Can you work these out from the model? Positions are in its coordinate system, mm. A direction names the side the tool comes from. Give positions to 0.01 mm unless a question says otherwise; leave off trailing zeros. Loops run counter-clockwise (first coordinate to the right, second up) from the corner with the lowest first, then second, coordinate; pieces in that order, holes last.
from build123d import *

# Parameters (mm, degrees)
SKETCH_1_R          = 30
SKETCH_1_R_2        = 15.5
EXTRUDE_1_DEPTH     = 8
SKETCH_2_R          = 21
CUT_EXTRUDE_1_DEPTH = 4
SKETCH_3_R          = 19
CUT_EXTRUDE_2_DEPTH = 1
SKETCH_4_R          = 2.25
CUT_EXTRUDE_3_DEPTH = 44.17406629
SKETCH_5_R          = 3.5
CUT_EXTRUDE_4_DEPTH = 4
CHAMFER_1_SIZE      = 1.414


with BuildPart() as part:
    # 草图1 → 拉伸1 (new body)
    with BuildSketch(Plane.XY):
        Circle(SKETCH_1_R)
        Circle(SKETCH_1_R_2, mode=Mode.SUBTRACT)
    extrude(amount=EXTRUDE_1_DEPTH)

    # 草图2 → 切除-拉伸1 (cut)
    with BuildSketch(Plane.XY.offset(8)):
        Circle(SKETCH_2_R)
    extrude(amount=-CUT_EXTRUDE_1_DEPTH, mode=Mode.SUBTRACT)

    # 草图3 → 切除-拉伸2 (cut)
    with BuildSketch(Plane.XY.offset(4)):
        Circle(SKETCH_3_R)
    extrude(amount=-CUT_EXTRUDE_2_DEPTH, mode=Mode.SUBTRACT)

    # 草图4 → 切除-拉伸3 (cut, through all)
    with BuildSketch(Plane(origin=(0, 0, 0), x_dir=(-1, 0, 0), z_dir=(0, 0, -1))):
        with Locations((12.5, 21.650635095)):
            Circle(SKETCH_4_R)
        with Locations((-12.5, 21.650635095)):
            Circle(SKETCH_4_R)
        with Locations((-25, 0)):
            Circle(SKETCH_4_R)
        with Locations((-12.5, -21.650635095)):
            Circle(SKETCH_4_R)
        with Locations((12.5, -21.650635095)):
            Circle(SKETCH_4_R)
        with Locations((25, 0)):
            Circle(SKETCH_4_R)
    extrude(amount=-CUT_EXTRUDE_3_DEPTH, mode=Mode.SUBTRACT)

    # 草图5 → 切除-拉伸4 (cut)
    with BuildSketch(Plane(origin=(0, 0, 0), x_dir=(-1, 0, 0), z_dir=(0, 0, -1))):
        with Locations((-12.5, 21.650635095)):
            Circle(SKETCH_5_R)
        with Locations((-25, 0)):
            Circle(SKETCH_5_R)
        with Locations((-12.5, -21.650635095)):
            Circle(SKETCH_5_R)
        with Locations((12.5, -21.650635095)):
            Circle(SKETCH_5_R)
        with Locations((25, 0)):
            Circle(SKETCH_5_R)
        with Locations((12.5, 21.650635095)):
            Circle(SKETCH_5_R)
    extrude(amount=-CUT_EXTRUDE_4_DEPTH, mode=Mode.SUBTRACT)

    # 倒角1
    chamfer_1_edges = [part.edges().sort_by_distance(p)[0] for p in [
        (-30, 0, 0),
    ]]
    chamfer(chamfer_1_edges, length=CHAMFER_1_SIZE)


solid = part.part
(1) Will these pins go through, and if not, where does the flat tip stop? P1, Ø3.5, axis at x = 11.5, y = 22.5, coming from the -Z side; P2, Ø2, axis at x = -14.5, z = 2, coming from the -Y side; P3, Ø4, axis at x = 12, z = 4.5, coming from the +Y side.
Returned:
P1: stops at z = 4
P2: stops at y = -26.79
P3: stops at y = 28.28
(2) Thinking about a two-plate mould opening in Y: for faces 4 (the cylindrical face through (12.79, -19.42, 5.97)), 5 (the flat face through (-16, -11, 4)), 6 (the flat face through (12, -12, 0)), 7 (the cylindrical face through (-29.97, 1.32, 4.66)), which applies, pulls with the +Y half, pulls with the -Y half, needs draft (parallel to the pull), parting line crosses it, or undercut?
Returned:
face 4: undercut
face 5: undercut
face 6: needs draft
face 7: parting line crosses it
(3) Suppose I cut it at A-A on y = 0. Give the number of separate pieces and of enclosed holes in the cut face, plus the area to 3 significant figures.
Returned:
separate pieces: 4
enclosed holes: 0
area: 87.0 mm2
(4) Suppose I cut it at B-B on x = 0. List the corners of the cut face in (y, z) for me, plus the area to 3 significant figures.
Returned:
outline: (-30, 1.41) - (-28.59, 0) - (-15.5, 0) - (-15.5, 3) - (-19, 3) - (-19, 4) - (-21, 4) - (-21, 8) - (-30, 8) - close; (15.5, 0) - (28.59, 0) - (30, 1.41) - (30, 8) - (21, 8) - (21, 4) - (19, 4) - (19, 3) - (15.5, 3) - close
area: 179 mm2
(5) Please list where these lines run through material, in increasing order: probe 1 along Y at (x, z) = (-9.5, 1.5); probe 2 along Y at (x, z) = (12.5, 2.5); probe 3 along X at (y, z) = (-23, 2.5).
Returned:
probe 1: y = -28.46 to -23.45, -19.85 to -12.25, 12.25 to 19.85, 23.45 to 28.46
probe 2: y = -27.27 to -25.15, -18.15 to -9.17, 9.17 to 18.15, 25.15 to 27.27
probe 3: x = -19.26 to -15.73, -9.27 to 9.27, 15.73 to 19.26
(6) Suppose I cut it at C-C on z = 4.75. List the corners of the cut face in (x, y) for me.
Returned:
outline: circle Ø60 at (0, 0); hole circle Ø4.5 at (-25, 0); hole circle Ø42 at (0, 0); hole circle Ø4.5 at (-12.5, -21.65); hole circle Ø4.5 at (-12.5, 21.65); hole circle Ø4.5 at (12.5, -21.65); hole circle Ø4.5 at (12.5, 21.65); hole circle Ø4.5 at (25, 0)
(7) Which directions (+Z, -Z, +X, -X, +Y, -Y) give clear straight access to the entire face, cutting with the end or side of a thin tool? Please do faces 1 (the cylindrical face through (-2.018, 15.368, 1.479)), 2 (the cylindrical face through (20.03, 6.31, 6.03)), 3 (the cylindrical face through (-28.34, 1.05, 1.97)).
Returned:
face 1: +Z, -Z
face 2: +Z
face 3: -Z
